Build history of the part. All positions in model axes, mm. Coordinates: 2 decimals unless noted, no trailing zeros. Order: outer loops, then holes, each group sorted by start corner. A loop starts at its lowest first (then second) coordinate and runs counter-clockwise, first axis right, second up. Notation, with made-up numbers: (76, -28) - (104, -28) arc R16 cw to (104, -18) - close; hole circle Ø8 at (36, 44). An arc over 180 degrees is marked (long way). Return JSON: item names as keys, results as strings.
from build123d import *

# Parameters (mm, degrees)
SKETCH1_R           = 3.1
BOSS_EXTRUDE1_DEPTH = 2
SKETCH2_R           = 5.75
CUT_EXTRUDE1_DEPTH  = 3


with BuildPart() as part:
    # Sketch1 → Boss-Extrude1 (new body)
    with BuildSketch(Plane(origin=(0, 0, 0), x_dir=(1, 0, 0), z_dir=(0, 1, 0))):
        with BuildLine():
            Line((-20, -30), (20, -30))
            ThreePointArc((20, -30), (27.071067812, -27.071067812), (30, -20))
            Line((30, -20), (30, 20))
            ThreePointArc((30, 20), (27.071067812, 27.071067812), (20, 30))
            Line((20, 30), (-20, 30))
            ThreePointArc((-20, 30), (-27.071067812, 27.071067812), (-30, 20))
            Line((-30, 20), (-30, -20))
            ThreePointArc((-30, -20), (-27.071067812, -27.071067812), (-20, -30))
        make_face()
        with Locations((-22.644230769, 22.644230769)):
            Circle(SKETCH1_R, mode=Mode.SUBTRACT)
        with Locations((-22.644230769, -22.644230769)):
            Circle(SKETCH1_R, mode=Mode.SUBTRACT)
        with Locations((22.644230769, -22.644230769)):
            Circle(SKETCH1_R, mode=Mode.SUBTRACT)
        with Locations((22.644230769, 22.644230769)):
            Circle(SKETCH1_R, mode=Mode.SUBTRACT)
    extrude(amount=BOSS_EXTRUDE1_DEPTH)

    # Sketch2 → Cut-Extrude1 (cut, through all)
    with BuildSketch(Plane(origin=(0, 2, 0), x_dir=(1, 0, 0), z_dir=(0, 1, 0))):
        Circle(SKETCH2_R)
    extrude(amount=-CUT_EXTRUDE1_DEPTH, mode=Mode.SUBTRACT)


solid = part.part
1. Cut at B-B on x = 0. Give the cut face in (y, z), plus the area to 3 significant figures.
Check values:
{"outline": "(0, -30) - (2, -30) - (2, -5.75) - (0, -5.75) - close; (0, 5.75) - (2, 5.75) - (2, 30) - (0, 30) - close", "area": "97.0 mm²"}
2. Probe L1, parallel to Z at x = -23.5, y = 0.75; L2, parallel to X at y = 0.4, z = 24.5; L3, parallel to X at y = 0.7, z = 22. List the from-to ranges inside material, lowest first.
Check values:
{"L1": "-29.37 to -25.62, -19.66 to 19.66, 25.62 to 29.37", "L2": "-28.93 to -25.13, -20.16 to 20.16, 25.13 to 28.93", "L3": "-29.8 to -25.68, -19.61 to 19.61, 25.68 to 29.8"}
3. Cut at C-C on y = 1.3. Give the cut face in (x, z), plus the area to 3 significant figures.
Check values:
{"outline": "(-30, -20) arc R10 ccw to (-20, -30) - (20, -30) arc R10 ccw to (30, -20) - (30, 20) arc R10 ccw to (20, 30) - (-20, 30) arc R10 ccw to (-30, 20) - close; hole circle Ø6.2 at (-22.64, -22.64); hole circle Ø6.2 at (-22.64, 22.64); hole circle Ø11.5 at (0, 0); hole circle Ø6.2 at (22.64, -22.64); hole circle Ø6.2 at (22.64, 22.64)", "area": "3,290 mm²"}
4. Mould opens along Z. For faces 1 (the cylindrical face through (-23.32, 0.99, -19.62)), 2 (the flat face through (0, 1, 30)), 3 (the cylindrical face through (-26.99, 0.99, -27.15)) say: pulls with the +Z half, pulls with the -Z half, needs draft (parallel to the pull), parting line crosses it, or undercut.
Check values:
{"face 1": "undercut", "face 2": "pulls with the +Z half", "face 3": "pulls with the -Z half"}
5. Cut at A-A on z = 0. Give the cut face in (x, y), plus the area to 3 significant figures.
Check values:
{"outline": "(-30, 0) - (-5.75, 0) - (-5.75, 2) - (-30, 2) - close; (5.75, 0) - (30, 0) - (30, 2) - (5.75, 2) - close", "area": "97.0 mm²"}
